Autodesk Inventor part; units mm, degrees
ref_plane "YZ Plane" through (0, 0, 0) normal (1, 0, 0) x (0, 1, 0)
ref_plane "XZ Plane" through (0, 0, 0) normal (0, 1, 0) x (-1, 0, 0)
ref_plane "XY Plane" through (0, 0, 0) normal (0, 0, 1) x (1, 0, 0)
sketch "Sketch1" plane through (0, 0, 0) normal (0, 0, 1) x (1, 0, 0)
  line L0 (9.75, 13) -> (7.875, 9.7524)
  line L1 (7.875, 9.7524) -> (4.125, 9.7524)
  line L2 (4.125, 9.7524) -> (2.25, 13)
  line L3 (2.25, 13) -> (4.125, 16.2476)
  line L4 (4.125, 16.2476) -> (7.875, 16.2476)
  line L5 (7.875, 16.2476) -> (9.75, 13)
  point P0 (0, 0)
  point P1 (6, 13)
  dimension "d0" = 7.5
extrude "Extrusion1" add sketch "Sketch1" along normal blind 18
sketch "Sketch2" plane through (4.125, 16.2476, 0) normal (0, 1, 0) x (1, 0, 0)
  line L0 (3.75, -18) -> (5.625, -18)
  line L1 (3.75, -18) -> (0, -18)
  line L2 (0, -18) -> (-5.625, -33.1757)
  line L3 (-1.875, 0) -> (-1.875, -18)
  line L4 (-5.625, -45.8247) -> (-5.625, -33.1757)
  line L5 (3.75, -18) -> (1.875, -18)
  line L6 (9.375, -45.8538) -> (9.375, -32.946)
  line L7 (9.375, -32.946) -> (3.75, -18)
  line L8 (9.375, -45.8538) -> (7.875, -45.8538)
  line L9 (7.875, -45.8538) -> (7.875, -33.2047)
  line L10 (-5.625, -45.8247) -> (-4.125, -45.8247)
  line L11 (-4.125, -45.8247) -> (-4.125, -33.4344)
  line L12 (2.1735, -18.0436) -> (2.158, -18)
  line L13 (1.875, -29) -> (6.2925, -29)
  line L14 (-2.4813, -29) -> (1.875, -29)
  line L15 (-4.125, -33.4344) -> (-2.4813, -29)
  line L16 (6.2925, -29) -> (7.875, -33.2047)
  line L17 (1.875, -18) -> (1.875, -45.8247)
  point P0 (-4.125, 0)
  dimension "d12" = 1.5
  dimension "d13" = 1.5
  dimension "d16" = 27.8247
  dimension "d17" = 11
  dimension "d21" = 12
extrude "Extrusion2" add sketch "Sketch2" against normal blind 6.5
sketch "Sketch3" plane through (-1.5, 9.7476, 33.1757) normal (-0.9377, 0, -0.3476) x (-0.3476, 0, 0.9377)
  point P0 (-31.6289, -9.7476)
sketch "Sketch5" plane through (4.125, 16.2476, 0) normal (0, 1, 0) x (1, 0, 0)
  line L0 (-1.875, -18) -> (0, -18)
  line L1 (-1.875, -18) -> (-1.875, -23.0586)
  line L2 (0, -18) -> (-5.625, -33.1757)
  line L3 (3.75, -18) -> (5.625, -18)
  line L4 (5.625, -18) -> (5.625, -22.982)
  line L5 (9.375, -32.946) -> (3.75, -18)
  point P0 (-4.125, 0)
extrude "Extrusion3" add sketch "Sketch5" against normal blind 6.5
sketch "Sketch6" plane through (13.5, 16.2476, 45.8538) normal (1, 0, 0) x (0, 0, -1)
  line L0 (0, 0) -> (0, -3.25)
  line L1 (0, 0) -> (0, -6.5)
  line L2 (0, -3.25) -> (6, -3.25)
  circle A0 centre (6, -3.25) radius 1.5
  point P0 (45.8538, -16.2476)
  dimension "d27" = 6
  dimension "d28" = 3
extrude "Extrusion4" cut sketch "Sketch6" against normal through all
properties part number "Test de pince"
Input: part model. Units: mm. Frame: model coordinates. A direction names the side the tool comes from. Give positions to 0.01 mm unless a question says otherwise; leave off trailing zeros. Loops run counter-clockwise (first coordinate to the right, second up) from the corner with the lowest first, then second, coordinate; pieces in that order, holes last. Notation, with made-up numbers: M 77.5,-40 L 116.5,-40 A29 cw 116.5,-14 Z; hole C -37.5,-4 d3. An arc over 180 degrees is marked long. Answer as CSV lines item,"result". Start each with the question number.
1. Line query: L1, parallel to X at y = 14.25, z = 43.5; L2, parallel to Z at x = 5.5, y = 15; L3, parallel to Y at x = 7.5, z = 14.5. Output: solid intervals per line, ascending.
2. Section C-C on z = 9.5. Return loops of the section in (x, y) (3 decimals), plus the area to 3 significant figures.
3. Pin query (flat end, axial travel): P1, Ø1.6, axis at x = -0.5, y = 12.5, coming from the +Z side; P2, Ø2, axis at y = 15, z = 21.5, coming from the +X side; P3, Ø3, axis at x = 6.5, z = 6.5, coming from the -Y side. Return the tip coordinate at first contact, or that it passes through.
4. Section B-B on y = 13.5. Return loops of the section in (x, z).
5. Pull-direction query (Z, two-part tool) for faces 6 (the face through (6, 13, 0)), 7 (the face through (13.5, 13, 38)), 8 (the face through (-0.739, 13.448, 38.423)); classes: released by +Z, released by -Z, zero draft, split by the parting line, or undercut.
6. Reachability of faces 1 (the face through (3.174, 14.601, 8.874)), 2 (the face through (8.826, 11.399, 8.874)), 3 (the face through (6, 13, 29)), 4 (the face through (8.799, 14.647, 8.874)), 5 (the face through (3.76, 10.06, 18)) from +Z, -Z, +X, -X, +Y, -Y: full face, straight path, thin tool, end or side. Return the list, or none.
7. Section A-A on z = 37. Return loops of the section in (x, y).
Computed values:
1,L1,"x = -1.5 to 0, 12 to 13.5"
1,L2,"z = 0 to 29"
1,L3,"y = 9.75 to 16.25"
2,outline,"M 2.25,13 L 4.125,9.752 L 7.875,9.752 L 9.75,13 L 7.875,16.248 L 4.125,16.248 Z"
2,area,"36.5 mm²"
3,P1,"stops at z = 45.82"
3,P2,"stops at x = 9.75"
3,P3,"stops at y = 9.75"
4,outline,"M -1.5,33.18 L 2.25,23.06 L 2.25,18 L 2.54,18 L 2.54,0 L 9.46,0 L 9.46,18 L 9.75,18 L 9.75,22.98 L 13.5,32.95 L 13.5,38.44 L 12,38.44 L 12,33.2 L 10.42,29 L 1.64,29 L 0,33.43 L 0,38.44 L -1.5,38.44 Z; M -1.5,41.27 L 0,41.27 L 0,45.82 L -1.5,45.82 Z; M 12,41.27 L 13.5,41.27 L 13.5,45.85 L 12,45.85 Z"
5,face 6,"released by -Z"
5,face 7,"zero draft"
5,face 8,"undercut"
6,face 1,"-Z, -X, +Y"
6,face 2,"-Z, +X, -Y"
6,face 3,"+Z, +Y, -Y"
6,face 4,"-Z, +X, +Y"
6,face 5,"-Z, -Y"
7,outline,"M -1.5,9.75 L 0,9.75 L 0,16.25 L -1.5,16.25 Z; M 12,9.75 L 13.5,9.75 L 13.5,16.25 L 12,16.25 Z"
